```python
from build123d import *

# Parameters (mm, degrees)
BOX063_W                   = 20
BOX063_H                   = 20
BOX063_DEPTH               = 2.5
SKETCH051_R                = 2.4
PAD018_DEPTH               = 2
CHAMFER003_SIZE            = 1.5
CHAMFER003_PLACEMENT_ANGLE = 180


with BuildPart() as cubo046:
    # Box063 → Box063 (new body)
    with BuildSketch(Plane.XY):
        with Locations((10, 10)):
            Rectangle(BOX063_W, BOX063_H)
    extrude(amount=BOX063_DEPTH)


with BuildPart() as pad018:
    # Pad018 base: copy of Cubo046
    add(cubo046.part)

    # Sketch051 → Pad018 (new body)
    with BuildSketch(Plane.XY.offset(2.5)):
        with Locations((10, 10.425099)):
            Circle(SKETCH051_R)
    extrude(amount=PAD018_DEPTH)


with BuildPart() as chamfer003:
    # Fusion039 base: copy of Cubo046
    add(cubo046.part)

    # Fusion039: union Pad018
    add(pad018.part)

    # Chamfer003
    chamfer003_edges = [chamfer003.edges().sort_by_distance(p)[0] for p in [
        (0, 0, 1.25),
        (0, 10, 0),
        (0, 20, 1.25),
        (10, 0, 0),
        (20, 0, 1.25),
        (10, 20, 0),
        (20, 20, 1.25),
        (20, 10, 0),
    ]]
    chamfer(chamfer003_edges, length=CHAMFER003_SIZE)


with BuildPart() as chamfer003_1:
    # Chamfer003 placement: moved
    add(chamfer003.part.moved(Location((-173, -157, 225.5))).rotate(Axis((-173, -157, 225.5), (1, 0, 0)), CHAMFER003_PLACEMENT_ANGLE))


solid = chamfer003_1.part
```
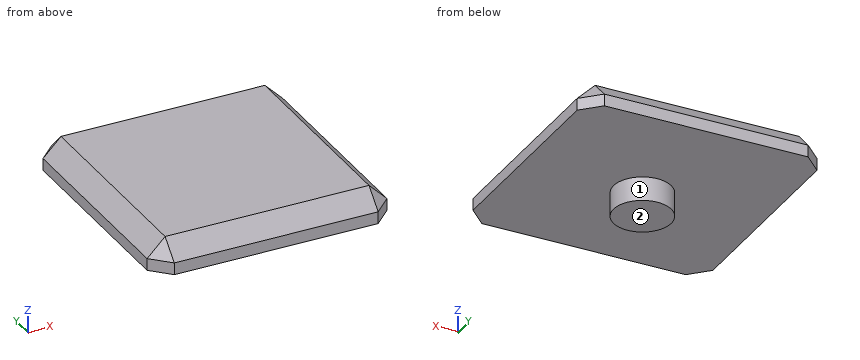
Here's how the part is built. I have some questions about the finished solid (model axes, mm). Face numbers are marked on the shaded views. A direction names the side the tool comes from. Round coordinates to 2 decimals unless told otherwise and drop trailing zeros. Write each loop counter-clockwise with the first axis right and the second up, starting at its lowest first coordinate (ties: lowest second). Pieces come first, ordered by that corner, then holes.
Q1. If we section it at B-B on y = -160.75: Write out the boundary of the cut face in (x, z).
Q2. If we section it at D-D on z = 222.5: Write out the boundary of the cut face in (x, y).
Q3. If we section it at C-C on x = -171.75: Write out the boundary of the cut face in (y, z), plus the area to 3 significant figures.
Q4. If we section it at A-A on x = -163: Write out the boundary of the cut face in (y, z).
Q5. Will these pins go through, and if not, where does the flat tip stop? P1, Ø3, axis at x = -159.5, y = -169.5, coming from the -Z side; P2, Ø1.5, axis at x = -163.5, z = 225, coming from the +Y side; P3, Ø2, axis at y = -173.5, z = 224.5, coming from the -X side.
Q6. Please list where these lines run through material, in increasing order: probe 1 along X at (y, z) = (-167.25, 222.15); probe 2 along Z at (x, y) = (-166.75, -160); probe 3 along Y at (x, z) = (-170.5, 224.65).
Q7. Which directions (+Z, -Z, +X, -X, +Y, -Y) give clear straight access to the entire face, cutting with the end or side of a thin tool? Please do the marked faces 1 and 2.
Answer below:
1. outline: (-173, 223) - (-153, 223) - (-153, 224) - (-154.5, 225.5) - (-171.5, 225.5) - (-173, 224) - close
2. outline: circle Ø4.8 at (-163, -167.43)
3. outline: (-176.75, 223) - (-157.25, 223) - (-157.25, 224) - (-158.5, 225.25) - (-175.5, 225.25) - (-176.75, 224) - close
3. area: 42.3 mm2
4. outline: (-177, 223) - (-169.83, 223) - (-169.83, 221) - (-165.03, 221) - (-165.03, 223) - (-157, 223) - (-157, 224) - (-158.5, 225.5) - (-175.5, 225.5) - (-177, 224) - close
5. P1: stops at z = 223
5. P2: stops at y = -157.25
5. P3: stops at x = -173
6. probe 1: x = -165.39 to -160.61
6. probe 2: z = 223 to 225.5
6. probe 3: y = -176.35 to -157.65
7. face 1: -Z
7. face 2: -Z, +X, -X, +Y, -Y
